from build123d import *
from build123d.topology import SkipClean

# Parameters (mm, degrees)
BOSS_EXTRUDE1_DEPTH = 6.35
SKETCH2_R           = 4.7625
CUT_EXTRUDE1_DEPTH  = 14.68691399
THREAD1_PITCH       = 1.5875


with BuildPart() as part:
    # Sketch1 → Boss-Extrude1 (new body)
    with BuildSketch(Plane(origin=(0, 0, 0), x_dir=(1, 0, 0), z_dir=(0, 1, 0))):
        Polygon((7.9375, -4.582717762), (7.9375, 4.582717762), (0, 9.165435523), (-7.9375, 4.582717762), (-7.9375, -4.582717762), (0, -9.165435523), align=None)
    extrude(amount=BOSS_EXTRUDE1_DEPTH)

    # Sketch2 → Cut-Extrude1 (cut, through all)
    with BuildSketch(Plane(origin=(0, 6.35, 0), x_dir=(1, 0, 0), z_dir=(0, 1, 0))):
        with Locations(Location((0, 0, 0), (0, 0, 270))):
            Circle(SKETCH2_R)
    extrude(amount=-CUT_EXTRUDE1_DEPTH, mode=Mode.SUBTRACT)

    # Thread1: the profile of Thread Profile1 profile screwed along a right-hand helix of 4 turns, 8 arcs to a turn; built about Z, then put on its axis
    with SkipClean():  # the faces are left unmerged after this step: merging them gives an invalid solid
        thread1_z = Axis((0, 0, 0), (0, 0, 1))
        thread1_corners = [(4.7628, 0, -0.000173205), (4.7628, 0, 1.389235701), (3.903240423, 0, 0.892968748), (3.903240423, 0, 0.496093748)]
        with BuildLine(mode=Mode.PRIVATE) as thread1_profile:
            Line(thread1_corners[0], thread1_corners[1])
            Line(thread1_corners[1], thread1_corners[2])
            Line(thread1_corners[2], thread1_corners[3])
            Line(thread1_corners[3], thread1_corners[0])
        thread1_cap = Face(thread1_profile.wire())
        thread1_turn_angles = [0, 22.5, 45, 67.5, 90, 112.5, 135, 157.5, 180, 202.5, 225, 247.5, 270, 292.5, 315, 337.5, 360]
        thread1_turn_weights = [1, 0.9238795325112867, 1, 0.9238795325112867, 1, 0.9238795325112867, 1, 0.9238795325112867, 1, 0.9238795325112867, 1, 0.9238795325112867, 1, 0.9238795325112867, 1, 0.9238795325112867, 1]
        thread1_turn_rails = [Edge.make_bspline([Vector(p[0], p[1], 0).rotate(thread1_z, thread1_turn_angles[k]) / thread1_turn_weights[k] + Vector(0, 0, p[2] + THREAD1_PITCH * thread1_turn_angles[k] / 360) for k in range(17)], [0, 0, 0, 1, 1, 2, 2, 3, 3, 4, 4, 5, 5, 6, 6, 7, 7, 8, 8, 8], 2, thread1_turn_weights) for p in thread1_corners]
        thread1_turn_sides = [Face.make_surface_from_curves(thread1_turn_rails[p[0]], thread1_turn_rails[p[1]]) for p in [(0, 1), (1, 2), (2, 3), (3, 0)]]
        thread1 = Plane(origin=(0, 6.35, 0), x_dir=(-1, 0, 0), z_dir=(0, -1, 0)) * Solid(Shell([*[p.moved(Location((0, 0, THREAD1_PITCH * i))) for i in range(4) for p in thread1_turn_sides], thread1_cap, thread1_cap.rotate(thread1_z, 1440).moved(Location((0, 0, THREAD1_PITCH * 1440 / 360)))]))
        add(thread1)


solid = part.part
Read the model definition and answer for the solid it produces. Units are mm, in the model's axes. A direction names the side the tool comes from. Coordinates: 2 decimals unless noted, no trailing zeros. Loops run counter-clockwise (first coordinate to the right, second up) from the corner with the lowest first, then second, coordinate; pieces in that order, holes last.
Q1. Consider probe 1 along Z at (x, y) = (-0.5, 5.75); probe 2 along Y at (x, z) = (3.5, -5); probe 3 along X at (y, z) = (5, 1.5). Determine where each line is inside the solid, lowest interval first.
Q2. Which of the six approach directions +Z, -Z, +X, -X, +Y, -Y give full straight-line access (tool end or side, diameter ignored) to faces 1 (the face through (-4.4, -0.7, 0)), 2 (the face through (-4.024, 3.131, 6.842))?
Q3. The mould has two halves that part along X. Classify faces 3 (the face through (3, 0, 4)), 4 (the face through (-3.91, 3.13, -6.91)), 5 (the face through (-4.4, 5.6, 0)): +X half, -X half, draft (parallel to the pull), parting line (faces both ways), or undercut.
Q4. The part is cut by section B-B on x = 6. Write down the section's boundary in (y, z), and give its area (3 significant figures).
Q5. The part is cut by section C-C on x = 4.25. Give the number of separate pieces and of enclosed holes in the cut face, and give its area (3 significant figures).
Q6. Each of these flat-tipped pins is pushed along its axis until it touches: pin 1 Ø0.7 at (x, y) = (-4.5, -0.5) entering from -Z; pin 2 Ø7.5 at (x, z) = (0, 0) entering from -Y; pin 3 Ø1.5 at (x, y) = (2, 5.5) entering from +Z; pin 4 Ø3 at (x, y) = (-6, 0.5) entering from -Z. Where does it stop, or does it pass through?
Q7. The part is cut by section A-A on z = 5. Write down the section's boundary in (x, y), and give its area (3 significant figures).
Results below:
1. probe 1: z = -8.88 to -4.33, 4.74 to 8.88
1. probe 2: y = 0 to 6.35
1. probe 3: x = -7.94 to -4.52, 3.67 to 7.94
2. face 1: -Z, -X, -Y
2. face 2: +Z, -X, +Y, -Y
3. face 3: draft
3. face 4: -X half
3. face 5: undercut
4. outline: (0, -5.7) - (6.35, -5.7) - (6.35, 5.7) - (0, 5.7) - close
4. area: 72.4 mm2
5. separate pieces: 1
5. enclosed holes: 3
5. area: 75.1 mm2
6. pin 1: stops at z = 0
6. pin 2: passes through
6. pin 3: stops at z = 8.44
6. pin 4: stops at z = -6.57
7. outline: (-7.21, 0) - (7.21, 0) - (7.21, 6.35) - (-7.21, 6.35) - close
7. area: 91.6 mm2
